Build history of the part. All positions in model axes, mm. Round coordinates to 2 decimals unless told otherwise and drop trailing zeros. Loops run counter-clockwise (first coordinate to the right, second up) from the corner with the lowest first, then second, coordinate; pieces in that order, holes last. Notation, with made-up numbers: M 32.5,-26.5 L 38.5,-26.5 A21 cw 38.5,12.5 Z; hole C 78,11.25 d9. An arc over 180 degrees is marked long. Write each question's results on one line, items separated by ' | '. Start each with the question number.
Autodesk Inventor part; units mm, degrees
ref_plane "YZ Plane" through (0, 0, 0) normal (1, 0, 0) x (0, 1, 0)
ref_plane "XZ Plane" through (0, 0, 0) normal (0, 1, 0) x (-1, 0, 0)
ref_plane "XY Plane" through (0, 0, 0) normal (0, 0, 1) x (1, 0, 0)
sketch "Sketch1" plane through (0, 0, 0) normal (0, 1, 0) x (-1, 0, 0)
  line L0 (0, 0) -> (101.6, 0)
  line L1 (101.6, 0) -> (101.6, -254)
  line L2 (101.6, -254) -> (0, -254)
  line L3 (0, -254) -> (0, 0)
  dimension "d0" = 254
  dimension "d1" = 101.6
extrude "Extrusion1" add sketch "Sketch1" along normal blind 3.175
sketch "Sketch2" plane through (-101.6, 0, 0) normal (0, 0, 1) x (1, 0, 0)
  line L0 (101.6, 3.175) -> (0, 3.175)
  line L1 (101.6, 0) -> (0, 0)
  line L2 (0, 3.175) -> (50.8, 3.175)
  line L3 (50.8, 3.175) -> (50.8, 0)
  line L4 (50.8, 0) -> (0, 0)
  line L5 (0, 0) -> (0, 3.175)
extrude "Extrusion2" add sketch "Sketch2" along normal blind 25.4
sketch "Sketch3" plane through (0, 3.175, 0) normal (0, 1, 0) x (1, 0, 0)
  circle A0 centre (-101.6, 254) radius 50.8
  point P0 (0, 0)
  dimension "d6" = 101.6
extrude "Extrusion3" cut sketch "Sketch3" against normal blind 25.4
sketch "Sketch4" plane through (-101.6, 0, -203.2) normal (-1, 0, 0) x (0, 0, 1)
  line L0 (203.2, 3.175) -> (-50.8, 3.175)
  line L1 (203.2, 0) -> (-0.4173, 0)
  line L2 (-0.4173, 0) -> (-0.4173, 3.175)
  line L3 (-0.4173, 3.175) -> (203.2, 3.175)
  line L4 (203.2, 3.175) -> (203.2, 0)
extrude "Extrusion4" add sketch "Sketch4" along normal blind 25.4
properties part number "Rotation Board"
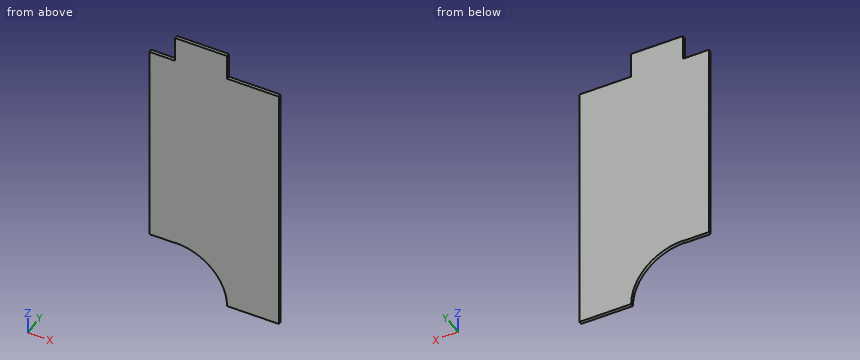
Item 1: Saw through at B-B, the plane x = -109. Give the cut face in (y, z) (3 decimals), then the cut area to 3 significant figures.
Item 2: Saw through at A-A, the plane y = 2.45. Give the cut face in (x, z).
Item 3: Saw through at C-C, the plane x = -71.5. Give the cut face in (y, z) (3 decimals), then the cut area to 3 significant figures.
Item 4: Drop flat-ended pins along their axis: pin 1 (2 mm diameter, centred on x = -109, z = -56, fed in from -Y); pin 2 (1 mm diameter, centred on x = -109.5, y = 1, fed in from +Z); pin 3 (1 mm diameter, centred on y = 1, z = 12.5, fed in from -X). Give the stop position or say it passes through.
Item 5: Drill centre lines: line 1 along Z through (x, y) = (-107, 0.65); line 2 along Z through (x, y) = (-16, 2.95); line 3 along X through (y, z) = (2.6, 5). Where is each one in solid material? Low to high. Write a range as [from, to].
Working result:
1) outline: M 0,-203.617 L 3.175,-203.617 L 3.175,0 L 0,0 Z | area: 646 mm²
2) outline: M -127,-203.62 L -101.6,-203.62 L -101.6,-203.2 A50.8 cw -50.8,-254 L 0,-254 L 0,0 L -50.8,0 L -50.8,25.4 L -101.6,25.4 L -101.6,0 L -127,0 Z
3) outline: M 0,-213.078 L 3.175,-213.078 L 3.175,25.4 L 0,25.4 Z | area: 757 mm²
4) pin 1: stops at y = 0 | pin 2: stops at z = 0 | pin 3: stops at x = -101.6
5) line 1: z = [-203.62, 0] | line 2: z = [-254, 0] | line 3: x = [-101.6, -50.8]
